```python
from build123d import *

# Parameters (mm, degrees)
F0_W     = 101.6
F0_H     = 355.6
F0_R     = 3.175
F0_R_2   = 9.525
F1_DEPTH = 12.7
F2_R     = 3.175
F3_DEPTH = 12.7


with BuildPart() as f1:
    # F0 (on Top) → F1 (new body)
    with BuildSketch(Plane.XY):
        with Locations((0, 47.119086)):
            Rectangle(F0_W, F0_H)
        with Locations((-25.4, -92.580914)):
            Circle(F0_R, mode=Mode.SUBTRACT)
        with Locations((0, 72.519086)):
            Circle(F0_R_2, mode=Mode.SUBTRACT)
    extrude(amount=F1_DEPTH)

    # F2 (on face) → F3 (cut)
    with BuildSketch(Plane(origin=(0, 224.919086, 0), x_dir=(-1, 0, 0), z_dir=(0, 1, 0))):
        with Locations((-25.4, 6.35)):
            Circle(F2_R)
        with Locations((0, 6.35)):
            Circle(F2_R)
        with Locations((25.4, 6.35)):
            Circle(F2_R)
    extrude(amount=-F3_DEPTH, mode=Mode.SUBTRACT)


solid = f1.part
```
Geometry check sheet. Reference: the model listing, model coordinates, mm. A direction names the side the tool comes from. Coordinates: 2 decimals unless noted, no trailing zeros. Order: outer loops, then holes, each group sorted by start corner. A loop starts at its lowest first (then second) coordinate and runs counter-clockwise, first axis right, second up. Notation, with made-up numbers: (4, 10.5) - (20, 10.5) arc R14 cw to (20, 29.5) - close; hole circle Ø9 at (60.25, 6). An arc over 180 degrees is marked (long way). Answer in a Markdown table with one row per item. Add a question column.
1. Section check A-A (x = -25.4). Enter the section's corners in (y, z) (3 decimals), plus the area to 3 significant figures.
2. Section check B-B (y = 78). Enter the section's corners in (x, z).
3. Gauge pin test, flat ends, axial feed: pin 1 Ø5 at (x, z) = (-25.4, 6.35) entering from +Y; pin 2 Ø5 at (x, y) = (7, 77) entering from +Z. Record the tip position at first contact, or that the pin passes through.
4. Material ranges on L1, parallel to Y at x = -25.4, z = 8; L2, parallel to X at y = 72.5, z = 6.5; L3, parallel to Y at x = -25.4, z = 2.75, recorded low to high. Write a range as [from, to].
5. Draft check along Z on faces 1 (the face through (-1.707, 218.658, 9.027)), 2 (the face through (-1, 50, 0)), 3 (the face through (-22.47, -93.8, 6.26)). Enter one of: +Z half, -Z half, draft (parallel to the pull), parting line (faces both ways), or undercut.
6. Section check D-D (x = 0). Enter the section's corners in (y, z) (3 decimals), plus the area to 3 significant figures.
7. Section check C-C (z = 6.35). Enter the section's corners in (x, y) (3 decimals), plus the area to 3 significant figures.
8. Access from +Z, -Z, +X, -X, +Y, -Y to the whole of each face (thin tool, end or side, straight path). Record for faces 4 (the face through (-1, 224.919, 10)), 5 (the face through (25, 212.219, 6)).
Data:
| question | item | result |
|---|---|---|
| 1 | outline | (-130.681, 0) - (-95.756, 0) - (-95.756, 12.7) - (-130.681, 12.7) - close; (-89.406, 0) - (224.919, 0) - (224.919, 3.175) - (212.219, 3.175) - (212.219, 9.525) - (224.919, 9.525) - (224.919, 12.7) - (-89.406, 12.7) - close |
| 1 | area | 4,350 mm² |
| 2 | outline | (-50.8, 0) - (-7.79, 0) - (-7.79, 12.7) - (-50.8, 12.7) - close; (7.79, 0) - (50.8, 0) - (50.8, 12.7) - (7.79, 12.7) - close |
| 3 | pin 1 | stops at y = 212.22 |
| 3 | pin 2 | stops at z = 12.7 |
| 4 | L1 | y = [-130.68, -95.76], [-89.41, 212.22] |
| 4 | L2 | x = [-50.8, -9.52], [9.52, 50.8] |
| 4 | L3 | y = [-130.68, -95.76], [-89.41, 224.92] |
| 5 | face 1 | undercut |
| 5 | face 2 | -Z half |
| 5 | face 3 | draft |
| 6 | outline | (-130.681, 0) - (62.994, 0) - (62.994, 12.7) - (-130.681, 12.7) - close; (82.044, 0) - (224.919, 0) - (224.919, 3.175) - (212.219, 3.175) - (212.219, 9.525) - (224.919, 9.525) - (224.919, 12.7) - (82.044, 12.7) - close |
| 6 | area | 4,190 mm² |
| 7 | outline | (-50.8, -130.681) - (50.8, -130.681) - (50.8, 224.919) - (28.575, 224.919) - (28.575, 212.219) - (22.225, 212.219) - (22.225, 224.919) - (3.175, 224.919) - (3.175, 212.219) - (-3.175, 212.219) - (-3.175, 224.919) - (-22.225, 224.919) - (-22.225, 212.219) - (-28.575, 212.219) - (-28.575, 224.919) - (-50.8, 224.919) - close; hole circle Ø6.35 at (-25.4, -92.581); hole circle Ø19.05 at (0, 72.519) |
| 7 | area | 35,600 mm² |
| 8 | face 4 | +Z, -Z, +X, -X, +Y |
| 8 | face 5 | +Y |
